```python
from build123d import *

# Parameters (mm, degrees)
SKETCH1_W           = 120
SKETCH1_H           = 30
SKETCH1_R           = 1.7
BOSS_EXTRUDE1_DEPTH = 30
SKETCH3_R           = 3
CUT_EXTRUDE1_DEPTH  = 30
CHAMFER1_SIZE       = 25


with BuildPart() as part:
    # Sketch1 → Boss-Extrude1 (new body)
    with BuildSketch(Plane.XY):
        Rectangle(SKETCH1_W, SKETCH1_H)
        with Locations((-40, 0)):
            Circle(SKETCH1_R, mode=Mode.SUBTRACT)
        with Locations((40, 0)):
            Circle(SKETCH1_R, mode=Mode.SUBTRACT)
    extrude(amount=-BOSS_EXTRUDE1_DEPTH)

    # Sketch3 → Cut-Extrude1 (cut)
    with BuildSketch(Plane(origin=(0, 0, -25), x_dir=(-1, 0, 0), z_dir=(0, 0, -1))):
        with Locations((-40, 0)):
            Circle(SKETCH3_R)
        with Locations((40, 0)):
            Circle(SKETCH3_R)
    extrude(amount=-CUT_EXTRUDE1_DEPTH, mode=Mode.SUBTRACT)

    # Chamfer1
    # the kernel refuses this chamfer: 25 mm, written as the material it takes off along each edge
    with BuildSketch(Plane(origin=(124.292074699, -15, 0), x_dir=(0, 0.9996219169112966, 0.02749587661058637), z_dir=(-1, 0, 0))) as chamfer1_piece_1:
        Polygon((CHAMFER1_SIZE * 0.999621916911, CHAMFER1_SIZE * 0.0274958766106), (-CHAMFER1_SIZE * 0.0274958766106, CHAMFER1_SIZE * 0.999621916911), (0, 0), align=None)
    extrude(amount=248.584149398, mode=Mode.SUBTRACT)


solid = part.part
```
Can you work these out from the model? Positions are in its coordinate system, mm. A direction names the side the tool comes from. Coordinates: 2 decimals unless noted, no trailing zeros. Loops run counter-clockwise (first coordinate to the right, second up) from the corner with the lowest first, then second, coordinate; pieces in that order, holes last.
1) Imagine slicing it at B-B on y = 0. List the corners of the cut face in (x, z) for me.
2) Which directions (+Z, -Z, +X, -X, +Y, -Y) give clear straight access to the entire face, cutting with the end or side of a thin tool? Please do faces 5 (the flat face through (-42, 0, -25)), 6 (the flat face through (60, 3, -18)).
3) Imagine slicing it at A-A on x = -40. List the corners of the cut face in (y, z) for me, plus the area to 4 significant figures.
4) Imagine slicing it at C-C on z = -4. List the corners of the cut face in (x, y) for me, plus the area to 3 significant figures.
5) I need wall thicknesses on probe 1 along X at (y, z) = (0, -21); probe 2 along Y at (x, z) = (-40, -27.4); probe 3 along Z at (x, y) = (-41, 7). Which ranges of each line are inside material? Lowest first, please.
6) Thinking about a two-plate mould opening in Y: for faces 1 (the flat face through (1, -2, -12)), 2 (the cylindrical face through (40, 3, -18)), 3 (the flat face through (-1, 0, -30)), 4 (the flat face through (-1, 15, -15)), which applies, pulls with the +Y half, pulls with the -Y half, needs draft (parallel to the pull), parting line crosses it, or undercut?
7) For pin 1 (1 mm diameter, centred on x = 8, y = 4, fed in from +Z); pin 2 (6.5 mm diameter, centred on x = 41, y = 0, fed in from +Z); pin 3 (3.5 mm diameter, centred on x = 40, y = 0, fed in from +Z), each with a flat end and sliding along its axis, tell me the tip position at first contact or that it passes through.
8) Imagine slicing it at D-D on x = -18. List the corners of the cut face in (y, z) for me.
Completed:
1. outline: (-60, -30) - (-41.7, -30) - (-41.7, -25) - (-43, -25) - (-43, -10) - (-60, -10) - close; (-38.3, -30) - (38.3, -30) - (38.3, -25) - (37, -25) - (37, -10) - (-37, -10) - (-37, -25) - (-38.3, -25) - close; (41.7, -30) - (60, -30) - (60, -10) - (43, -10) - (43, -25) - (41.7, -25) - close
2. face 5: +Z
2. face 6: +Z, -Z, +X, +Y, -Y
3. outline: (-15, -30) - (-1.7, -30) - (-1.7, -25) - (-3, -25) - (-3, -13) - (-15, -25) - close; (1.7, -30) - (15, -30) - (15, 0) - (10, 0) - (3, -7) - (3, -25) - (1.7, -25) - close
3. area: 480.5 mm2
4. outline: (-60, 6) - (60, 6) - (60, 15) - (-60, 15) - close
4. area: 1,080 mm2
5. probe 1: x = -60 to -43, -37 to 37, 43 to 60
5. probe 2: y = -15 to -1.7, 1.7 to 15
5. probe 3: z = -30 to -3
6. face 1: pulls with the -Y half
6. face 2: undercut
6. face 3: needs draft
6. face 4: pulls with the +Y half
7. pin 1: stops at z = -5.5
7. pin 2: stops at z = -6.75
7. pin 3: stops at z = -25
8. outline: (-15, -30) - (15, -30) - (15, 0) - (10, 0) - (-15, -25) - close
